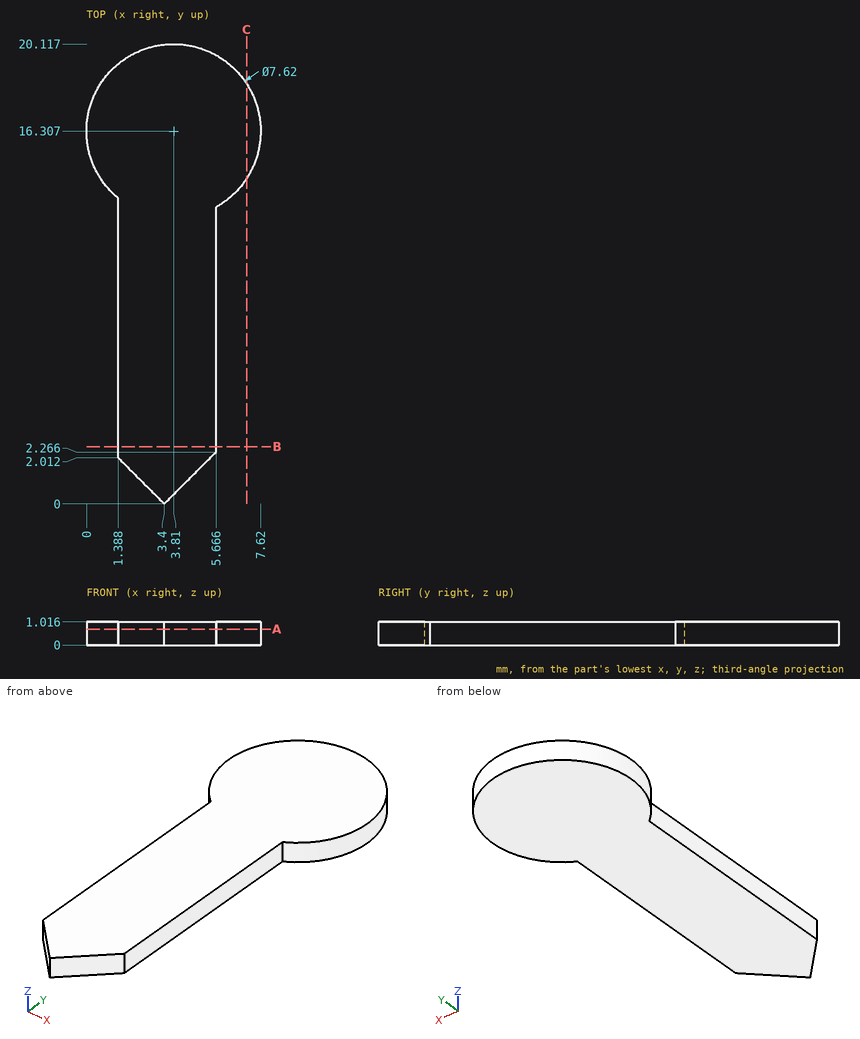
Geometry: see drawing. Coordinates: mm, zero at the bounding-box minimum. Coordinates: 2 decimals unless noted, no trailing zeros. Loops run counter-clockwise (first coordinate to the right, second up) from the corner with the lowest first, then second, coordinate; pieces in that order, holes last. Notation, with made-up numbers: (43.5, -13) -> (102.5, -13) arc R23 cw to (102.5, 13) -> close; hole circle Ø4 at (-24.75, 77). An arc over 180 degrees is marked (long way). Use a Markdown table: item, result.
1) Material intervals for line 1 along X through (y, z) = (6.5, 0.1); line 2 along X through (y, z) = (16.5, 0.85) (1 decimal); line 3 along Y through (x, z) = (3, 0.95), sorted ascending. Write a range as from..to.
Results found:
| item | result |
|---|---|
| line 1 | x = 1.39..5.67 |
| line 2 | x = 0..7.6 |
| line 3 | y = 0.4..20.03 |
2) Cut plane A-A (z = 0.7). Return the cut outline in (x, y).
Results found:
| item | result |
|---|---|
| outline | (1.39, 2.01) -> (3.4, 0) -> (5.67, 2.27) -> (5.67, 12.98) arc R3.81 ccw (long way) to (1.39, 13.37) -> close |
3) Cut plane C-C (x = 7). Return the cut outline in (y, z).
Results found:
| item | result |
|---|---|
| outline | (14.22, 0) -> (18.39, 0) -> (18.39, 1.02) -> (14.22, 1.02) -> close |
4) Cut plane B-B (y = 2.5). Return the cut outline in (x, z).
Results found:
| item | result |
|---|---|
| outline | (1.39, 0) -> (5.67, 0) -> (5.67, 1.02) -> (1.39, 1.02) -> close |
